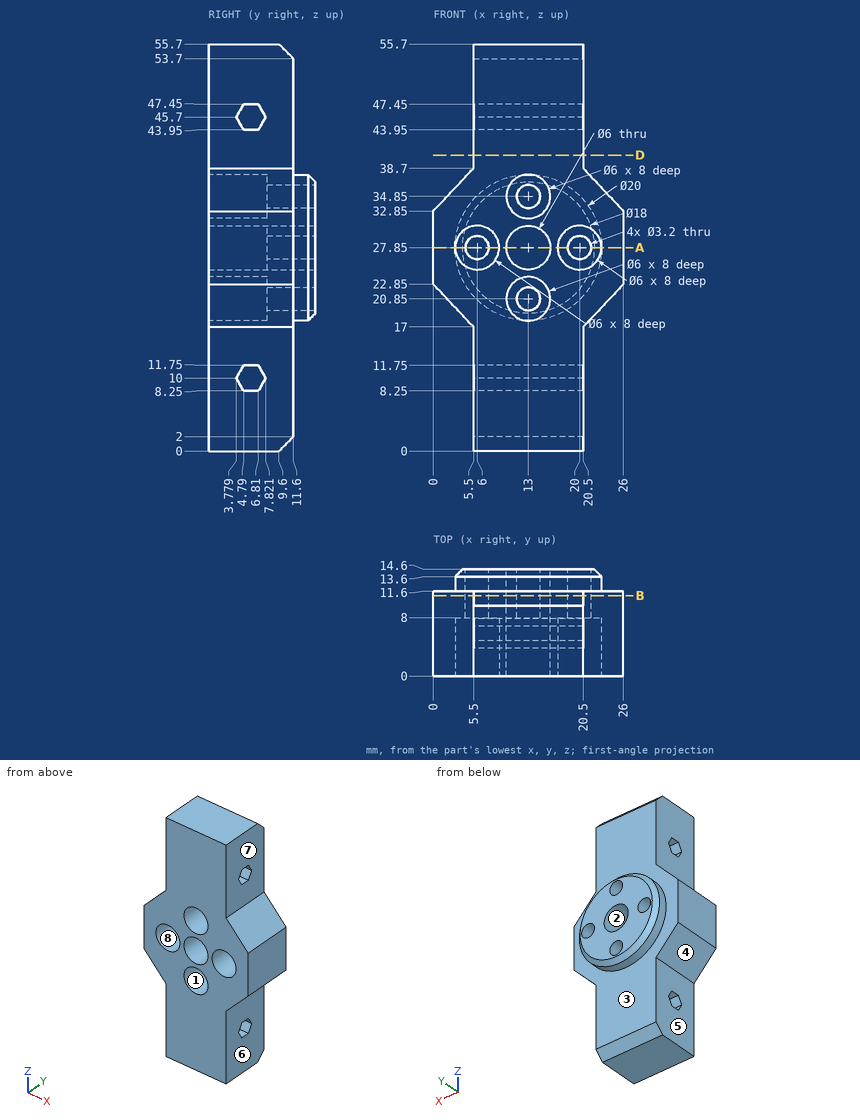
Can you work these out from the drawing? Everything is in mm from the part's minimum corner. A direction names the side the tool comes from. Coordinates: 2 decimals unless noted, no trailing zeros. Order: outer loops, then holes, each group sorted by start corner. A loop starts at its lowest first (then second) coordinate and runs counter-clockwise, first axis right, second up. Notation, with made-up numbers: M 12,30.25 L 23,30.25 A16 ccw 23,39.25 Z; hole C -7,87.5 d11. An arc over 180 degrees is marked long. Answer as CSV lines item,"result". Start each with the question number.
1. I want a section at B-B, the plane y = 11. Write out the boundary of the cut face in (x, z).
2. For pin 1 (1 mm diameter, centred on x = 10, z = 42, fed in from +Y); pin 2 (1 mm diameter, centred on y = 10.5, z = 47, fed in from +X); pin 3 (3 mm diameter, centred on x = 13, z = 22, fed in from -Y), each with a flat end and sliding along its axis, tell me the tip position at first contact or that it passes through.
3. I want a section at D-D, the plane z = 40.5. Write out the boundary of the cut face in (x, y).
4. We'd pull the mould along X, two halves only. Please class the marked faces 1, 2, 3 and 4: released by +X, released by -X, zero draft, split by the parting line, or undercut.
5. I need wall thicknesses on line 1 (X direction, y = 12.75, z = 27.85); line 2 (X direction, y = 6, z = 27.85); line 3 (Z direction, x = 13, y = 3.5). Which ranges of each line are inside material? Lowest first, please. Write a range as [from, to].
6. On a 3-axis mill with a long thin cutter (end or side, diameter ignored), from which of +Z, -Z, +X, -X, +Y, -Y can I reach the whole of each face in a straight line? I mean the marked faces 5, 6, 7 and 8. Say none if no direction works.
7. I want a section at A-A, the plane z = 27.85. Count the separate pieces of the cut face and the enclosed holes in it, and give its area (3 significant figures).
Recorded:
1,outline,"M 0,22.85 L 5.5,17 L 5.5,1.4 L 20.5,1.4 L 20.5,17 L 26,22.85 L 26,32.85 L 20.5,38.7 L 20.5,54.3 L 5.5,54.3 L 5.5,38.7 L 0,32.85 Z; hole C 6,27.85 d3.2; hole C 13,27.85 d6; hole C 13,20.85 d3.2; hole C 13,34.85 d3.2; hole C 20,27.85 d3.2"
2,pin 1,"stops at y = 11.6"
2,pin 2,"stops at x = 20.5"
2,pin 3,"stops at y = 8"
3,outline,"M 5.5,0 L 20.5,0 L 20.5,11.6 L 5.5,11.6 Z"
4,face 1,"undercut"
4,face 2,"undercut"
4,face 3,"zero draft"
4,face 4,"released by -X"
5,line 1,"x = [3, 4.4], [7.6, 10], [16, 18.4], [21.6, 23]"
5,line 2,"x = [0, 3], [9, 10], [16, 17], [23, 26]"
5,line 3,"z = [0, 17.85], [23.85, 24.85], [30.85, 31.85], [37.85, 55.7]"
6,face 5,"-Z, -X, +Y, -Y"
6,face 6,"-Z, +X, +Y, -Y"
6,face 7,"+Z, +X, +Y, -Y"
6,face 8,"-Y"
7,separate pieces,"4"
7,enclosed holes,"0"
7,area,"135 mm2"
